CAD build for the part. Positions are in the model's coordinates, mm. A direction names the side the tool comes from. Give positions to 0.01 mm unless a question says otherwise; leave off trailing zeros. Loops run counter-clockwise (first coordinate to the right, second up) from the corner with the lowest first, then second, coordinate; pieces in that order, holes last.
```python
from build123d import *

# Parameters (mm, degrees)
SKETCH1_R                                    = 18.669
SKETCH1_R_2                                  = 5.715
NUT_BODY_EXTRUDE_DEPTH                       = 25.4
SKETCH2_R                                    = 18.669
SKETCH2_W                                    = 31.75
SKETCH2_H                                    = 19.05
NUT_TRIM_CUT_EXTRUDE_DEPTH                   = 37.636363384
CBORE_FOR_10_SOCKET_HEAD_CAP_SCREW1_AT_COUNT = 2
CBORE_FOR_10_SOCKET_HEAD_CAP_SCREW1_AT_PITCH = 12.7
CBORE_FOR_10_SOCKET_HEAD_CAP_SCREW1_2_COUNT  = 2
CBORE_FOR_10_SOCKET_HEAD_CAP_SCREW1_2_PITCH  = 27.268056403
CBORE_FOR_10_SOCKET_HEAD_CAP_SCREW1_3_COUNT  = 2
CBORE_FOR_10_SOCKET_HEAD_CAP_SCREW1_3_PITCH  = 24.13


with BuildPart() as part:
    # Sketch1 → nut-body-extrude (new body)
    with BuildSketch(Plane.XY):
        Circle(SKETCH1_R)
        Circle(SKETCH1_R_2, mode=Mode.SUBTRACT)
    extrude(amount=NUT_BODY_EXTRUDE_DEPTH)

    # Sketch2 → nut-trim-cut-extrude (cut, through all)
    with BuildSketch(Plane.XY):
        Circle(SKETCH2_R)
        Rectangle(SKETCH2_W, SKETCH2_H, mode=Mode.SUBTRACT)
    extrude(amount=NUT_TRIM_CUT_EXTRUDE_DEPTH, mode=Mode.SUBTRACT)

    # Sketch4 → CBORE for #10 Socket Head Cap Screw1 (revolve, cut)
    with BuildSketch(Plane(origin=(12.065, 9.525, 6.35), x_dir=(0, 0, 1), z_dir=(1, 0, 0))):
        Polygon((0, 0), (0, 19.05), (2.5527, 19.05), (2.5527, 4.826), (4.191, 4.826), (4.191, 0.635), (4.826, 0), align=None)
    cbore_for_10_socket_head_cap_screw1 = revolve(axis=Axis((12.065, 15.875, 6.35), (0, -1, 0)), mode=Mode.SUBTRACT)

    # CBORE for #10 Socket Head Cap Screw1 at: CBORE for #10 Socket Head Cap Screw1 ×2
    with Locations(*[(0, 0, i * CBORE_FOR_10_SOCKET_HEAD_CAP_SCREW1_AT_PITCH) for i in range(1, CBORE_FOR_10_SOCKET_HEAD_CAP_SCREW1_AT_COUNT)]):
        add(cbore_for_10_socket_head_cap_screw1, mode=Mode.SUBTRACT)

    # CBORE for _10 Socket Head Cap Screw1 2: CBORE for #10 Socket Head Cap Screw1 ×2
    with Locations(*[Vector(-0.8849182223819826, 0, 0.46574643283262207) * (i * CBORE_FOR_10_SOCKET_HEAD_CAP_SCREW1_2_PITCH) for i in range(1, CBORE_FOR_10_SOCKET_HEAD_CAP_SCREW1_2_COUNT)]):
        add(cbore_for_10_socket_head_cap_screw1, mode=Mode.SUBTRACT)

    # CBORE for _10 Socket Head Cap Screw1 3: CBORE for #10 Socket Head Cap Screw1 ×2
    with Locations(*[(-i * CBORE_FOR_10_SOCKET_HEAD_CAP_SCREW1_3_PITCH, 0, 0) for i in range(1, CBORE_FOR_10_SOCKET_HEAD_CAP_SCREW1_3_COUNT)]):
        add(cbore_for_10_socket_head_cap_screw1, mode=Mode.SUBTRACT)


solid = part.part
```
1. Probe line 1 along X through (y, z) = (-5.75, 6.5) (3 decimals); line 2 along Z through (x, y) = (11, -1); line 3 along Z through (x, y) = (-14, -1.75). List the from-to ranges inside material, lowest first.
Responses:
line 1: x = -15.875 to -14.613, -9.517 to 9.517, 14.613 to 15.875
line 2: z = 0 to 4.03, 8.67 to 16.73, 21.37 to 25.4
line 3: z = 0 to 4.69, 8.01 to 17.39, 20.71 to 25.4
2. Pull direction X, two halves, no side cores. Call faces 3 (the face through (15.875, 0, 13)), 4 (the face through (0, -9.525, 13)), 5 (the face through (7.767, 9, 6.513)), 6 (the face through (-9, 4.699, 6)): released by +X, released by -X, zero draft, split by the parting line, or undercut.
Responses:
face 3: released by +X
face 4: zero draft
face 5: undercut
face 6: undercut
3. Drop flat-ended pins along their axis: pin 1 (9.5 mm diameter, centred on x = 12.065, z = 6.35, fed in from +Y); pin 2 (6.5 mm diameter, centred on x = 12.065, z = 19.05, fed in from +Y); pin 3 (6.5 mm diameter, centred on x = 13, z = 19.5, fed in from +Y). Give the stop position or say it passes through.
Responses:
pin 1: stops at y = 9.45
pin 2: stops at y = 4.7
pin 3: stops at y = 8.99
4. Saw through at D-D, the plane z = 12.5. List the corners of the cut face in (x, y) (3 decimals).
Responses:
outline: (-15.875, -9.525) - (15.875, -9.525) - (15.875, 9.525) - (-15.875, 9.525) - close; hole circle Ø11.43 at (0, 0)
5. Saw through at B-B, the plane x = 0. List the corners of the cut face in (y, z) (3 decimals), and give its area (3 significant figures).
Responses:
outline: (-9.525, 0) - (-5.715, 0) - (-5.715, 25.4) - (-9.525, 25.4) - close; (5.715, 0) - (9.525, 0) - (9.525, 25.4) - (5.715, 25.4) - close
area: 194 mm2
6. Saw through at C-C, the plane y = 0. List the corners of the cut face in (x, z) (3 decimals).
Responses:
outline: (-15.875, 0) - (-5.715, 0) - (-5.715, 25.4) - (-15.875, 25.4) - close; (5.715, 0) - (15.875, 0) - (15.875, 25.4) - (5.715, 25.4) - close; hole circle Ø5.105 at (-12.065, 6.35); hole circle Ø5.105 at (-12.065, 19.05); hole circle Ø5.105 at (12.065, 6.35); hole circle Ø5.105 at (12.065, 19.05)
7. Saw through at A-A, the plane z = 6.35. List the corners of the cut face in (x, y) (3 decimals).
Responses:
outline: (-15.875, -9.525) - (-14.618, -9.525) - (-14.618, 4.699) - (-15.875, 4.699) - close; (-9.512, -9.525) - (9.512, -9.525) - (9.512, 4.699) - (7.874, 4.699) - (7.874, 8.89) - (7.239, 9.525) - (-7.239, 9.525) - (-7.874, 8.89) - (-7.874, 4.699) - (-9.512, 4.699) - close; (14.618, -9.525) - (15.875, -9.525) - (15.875, 4.699) - (14.618, 4.699) - close; hole circle Ø11.43 at (0, 0)
8. Tool access for faces 1 (the face through (5.45, 1.72, 12.52)), 2 (the face through (7.877, 6.824, 19.209)): list every direction of +Z, -Z, +X, -X, +Y, -Y with a clear straight run to the whole face (end or side of a thin tool).
Responses:
face 1: +Z, -Z
face 2: +Y
